Can you work these out from the model? Positions are in its coordinate system, mm. A direction names the side the tool comes from. Give positions to 0.01 mm unless a question says otherwise; leave off trailing zeros. Order: outer loops, then holes, each group sorted by start corner. A loop starts at its lowest first (then second) coordinate and runs counter-clockwise, first axis right, second up. Notation, with made-up numbers: (-33.75, 19.5) - (-7.75, 19.5) arc R30 ccw to (-7.75, 56.5) - close; hole circle Ø2 at (-32, 51.25). An arc over 180 degrees is marked (long way). Write each question's results on one line, items separated by ' | '. Start each with the question number.
Autodesk Inventor part; units mm, degrees
ref_plane "Work Plane1" through (-15, 0, 0) normal (1, 0, 0) x (0, 1, 0)
ref_plane "Work Plane2" through (-3, 0, 0) normal (1, 0, 0) x (0, 1, 0)
ref_plane "XZ Plane" through (0, 0, 0) normal (0, 1, 0) x (-1, 0, 0)
ref_plane "Work Plane1" through (-15, 0, 0) normal (1, 0, 0) x (0, 1, 0)
sketch "Sketch1" plane through (-15, 0, 0) normal (1, 0, 0) x (0, 1, 0)
  line L0 (0, 20) -> (0, 0)
  arc A0 (15, 20.245) -> (4.7085, 20) centre (10, 14) ccw
  line L1 (15, 0) -> (15, 20.245)
  line L2 (15, 0) -> (0, 0)
  line L3 (4.7085, 20) -> (0, 20)
extrude "Extrusion8" add sketch "Sketch1" along normal blind 30
sketch "Sketch2" plane through (15, 0, 0) normal (1, 0, 0) x (0, 0, -1)
  line L0 (-20.245, 15) -> (0, 15)
  line L1 (-20, 4) -> (-20, 4.7085)
  line L2 (0, 4) -> (0, 15)
  arc A0 (-20.245, 15) -> (-20, 4.7085) centre (-14, 10) ccw
  line L3 (-20, 4) -> (0, 4)
extrude "Extrusion7" cut sketch "Sketch2" against normal blind 8
sketch "Sketch3" plane through (-15, 0, 0) normal (1, 0, 0) x (0, 1, 0)
  line L0 (4.7085, 20) -> (4, 20)
  line L1 (15, 20.245) -> (15, 0)
  line L2 (4, 20) -> (4, 0)
  arc A0 (15, 20.245) -> (4.7085, 20) centre (10, 14) ccw
  line L3 (15, 0) -> (4, 0)
extrude "Extrusion6" cut sketch "Sketch3" along normal blind 8
ref_plane "Work Plane2" through (-3, 0, 0) normal (1, 0, 0) x (0, 1, 0)
sketch "Sketch4" plane through (-3, 0, 0) normal (1, 0, 0) x (0, 1, 0)
  arc A0 (15, 20.245) -> (4.7085, 20) centre (10, 14) ccw
  arc A1 (1, 14) -> (4, 7.2918) centre (10, 14) ccw
  line L0 (15, 20.245) -> (15, 0)
  line L1 (4.7085, 20) -> (1, 20)
  line L2 (4, 7.2918) -> (4, 0)
  line L3 (1, 20) -> (1, 14)
  line L4 (15, 0) -> (4, 0)
extrude "Extrusion5" cut sketch "Sketch4" along normal blind 6
sketch "Sketch5" plane through (-3, 4, 7.2918) normal (0, 1, 0) x (1, 0, 0)
  arc A0 (-6.409, -0.2992) -> (-9.591, -0.2992) centre (-8, 1.2918) ccw
  line L0 (-8, -1.8902) -> (-6.409, -0.2992)
  line L1 (-9.591, -0.2992) -> (-8, -1.8902)
extrude "Extrusion4" cut sketch "Sketch5" against normal blind 4
sketch "Sketch6" plane through (0, 0, 0) normal (0, 1, 0) x (-1, 0, 0)
  line L0 (-9.409, 7.591) -> (-11, 9.182)
  arc A0 (-12.591, 7.591) -> (-9.409, 7.591) centre (-11, 6) ccw
  line L1 (-11, 9.182) -> (-12.591, 7.591)
extrude "Extrusion3" cut sketch "Sketch6" along normal blind 4
sketch "Sketch7" plane through (7, 0, 0) normal (1, 0, 0) x (0, 0, -1)
  arc A0 (-15.591, 8.409) -> (-15.591, 11.591) centre (-14, 10) ccw
  line L0 (-17.182, 10) -> (-15.591, 8.409)
  line L1 (-15.591, 11.591) -> (-17.182, 10)
extrude "Extrusion2" cut sketch "Sketch7" against normal blind 4
sketch "Sketch8" plane through (-3, 0, 0) normal (1, 0, 0) x (0, 1, 0)
  arc A0 (8.409, 15.591) -> (11.591, 15.591) centre (10, 14) ccw
  line L0 (8.409, 15.591) -> (10, 17.182)
  line L1 (10, 17.182) -> (11.591, 15.591)
extrude "Extrusion1" cut sketch "Sketch8" against normal blind 4 draft 0
properties part number "Y-axis Belt Return" material "ASA Plastic"
Q1. If we section it at B-B (x = 3.75): Please give me the cut outline in (y, z) (1 decimal).
Q2. Will these pins go through, and if not, where does the flat tip stop? P1, Ø6.5, axis at x = 12.5, z = 13, coming from the +Y side; P2, Ø5, axis at x = 4, y = 2.5, coming from the +Z side (3 decimals); P3, Ø6, axis at y = 10, z = 14, coming from the +X side.
Q3. If I drill on probe 1 along X at (y, z) = (1.55, 6); probe 2 along X at (y, z) = (13.75, 19); probe 3 along X at (y, z) = (2.75, 12.5), over which ranges is the centre line in solid material (lowest first)? Write a range as from..to.
Q4. If we section it at D-D (y = 8.75): Please give me the cut outline in (x, z).
Q5. If we section it at A-A (z = 18.25): Please give me the cut outline in (x, y), plus the area to 3 significant figures.
Q6. Which directions (+Z, -Z, +X, -X, +Y, -Y) give clear straight access to the entire face, cutting with the end or side of a thin tool? Please do faces 4 (the flat face through (11.78, 1.97, 8.4)), 5 (the flat face through (-3, 8, 11)), 6 (the flat face through (11, 4, 10)), 7 (the flat face through (-7, 9, 11)), 8 (the flat face through (5.028, 10.807, 16.375)).
Q7. Thinking about a two-plate mould opening in Z: for faces 1 (the flat face through (-0.2, 0.8, 20)), 2 (the flat face through (5.03, 9.22, 16.4)), 3 (the flat face through (5, 15, 10)), which applies, released by +Z, released by -Z, zero draft, split by the parting line, or undercut?
Q8. If we section it at C-C (z = 6.5): Please give me the cut outline in (x, y), plus the area to 3 significant figures.
Findings below:
1) outline: (0, 0) - (15, 0) - (15, 20.2) arc R8 ccw to (4.7, 20) - (0, 20) - close; hole (8.4, 15.6) arc R2.3 ccw (long way) to (11.6, 15.6) - (10, 17.2) - close
2) P1: stops at y = 4 | P2: stops at z = 20.245 | P3: stops at x = 7
3) probe 1: x = -15..-13.25, -8.75..8.75, 13.25..15 | probe 2: x = -7..-3, 3..7 | probe 3: x = -15..-3, 3..15
4) outline: (-7, 0) - (-3, 0) - (-3, 12.13) - (-7, 12.13) - close; (-7, 15.93) - (-3, 15.93) - (-3, 21.9) - (-7, 21.9) - close; (3, 0) - (7, 0) - (7, 12.13) - (3, 12.13) - close; (3, 15.93) - (7, 15.93) - (7, 21.9) - (3, 21.9) - close
5) outline: (-15, 0) - (15, 0) - (15, 4) - (7, 4) - (7, 15) - (3, 15) - (3, 1) - (-3, 1) - (-3, 15) - (-7, 15) - (-7, 4) - (-15, 4) - close | area: 190 mm2
6) face 4: +Y, -Y | face 5: +Z, +Y | face 6: +Z, -Z, +X, +Y | face 7: +Z, -Z, -X, +Y | face 8: +X, -X
7) face 1: released by +Z | face 2: undercut | face 3: zero draft
8) outline: (-15, 0) - (-13.19, 0) - (-13.19, 4) - (-15, 4) - close; (-8.81, 0) - (8.81, 0) - (8.81, 4) - (7, 4) - (7, 15) - (3, 15) - (3, 4) - (-3, 4) - (-3, 15) - (-7, 15) - (-7, 4) - (-8.81, 4) - close; (13.19, 0) - (15, 0) - (15, 4) - (13.19, 4) - close | area: 173 mm2
